For this review, take the finished solid that the model builds, in its own axes (mm). Give positions to 0.01 mm unless a question says otherwise; leave off trailing zeros. Write each loop counter-clockwise with the first axis right and the second up, starting at its lowest first coordinate (ties: lowest second). Pieces come first, ordered by that corner, then holes. Notation, with made-up numbers: M 54.5,60 L 75.5,60 A28 ccw 75.5,87 Z; hole C -6,17.25 d2. An arc over 180 degrees is marked long. Write item = value, one per line.
```python
from build123d import *

# Parameters (mm, degrees)
SKETCH1_R           = 3
SKETCH1_R_2         = 1.5
BOSS_EXTRUDE1_DEPTH = 4


with BuildPart() as part:
    # Sketch1 → Boss-Extrude1 (new body)
    with BuildSketch(Plane.XY):
        with BuildLine():
            Line((2, 13), (2.375498971, 4.399659605))
            ThreePointArc((2.375498971, 4.399659605), (3.535533906, 3.535533906), (4.399659605, 2.375498971))
            Line((4.399659605, 2.375498971), (13, 2))
            ThreePointArc((13, 2), (15, 0), (13, -2))
            Line((13, -2), (4.399659605, -2.375498971))
            ThreePointArc((4.399659605, -2.375498971), (3.535533906, -3.535533906), (2.375498971, -4.399659605))
            Line((2.375498971, -4.399659605), (2, -13))
            ThreePointArc((2, -13), (0, -15), (-2, -13))
            Line((-2, -13), (-2.375498971, -4.399659605))
            ThreePointArc((-2.375498971, -4.399659605), (-3.535533906, -3.535533906), (-4.399659605, -2.375498971))
            Line((-4.399659605, -2.375498971), (-13, -2))
            ThreePointArc((-13, -2), (-15, 0), (-13, 2))
            Line((-13, 2), (-4.399659605, 2.375498971))
            ThreePointArc((-4.399659605, 2.375498971), (-3.535533906, 3.535533906), (-2.375498971, 4.399659605))
            Line((-2.375498971, 4.399659605), (-2, 13))
            ThreePointArc((-2, 13), (0, 15), (2, 13))
        make_face()
        Circle(SKETCH1_R, mode=Mode.SUBTRACT)
        with Locations((0, 13)):
            Circle(SKETCH1_R_2, mode=Mode.SUBTRACT)
        with Locations((13, 0)):
            Circle(SKETCH1_R_2, mode=Mode.SUBTRACT)
        with Locations((0, -13)):
            Circle(SKETCH1_R_2, mode=Mode.SUBTRACT)
        with Locations((-13, 0)):
            Circle(SKETCH1_R_2, mode=Mode.SUBTRACT)
    extrude(amount=BOSS_EXTRUDE1_DEPTH)


solid = part.part
```
1. For line 1 along Y through (x, z) = (0, 3); line 2 along Y through (x, z) = (13, 3.15); line 3 along X through (y, z) = (-0.75, 2.55), list the stretches that pass through material, from the lowest coordinate up. Write a range as from..to.
Responses:
line_1 = -15..-14.5, -11.5..-3, 3..11.5, 14.5..15
line_2 = -2..-1.5, 1.5..2
line_3 = -14.85..-14.3, -11.7..-2.9, 2.9..11.7, 14.3..14.85
2. We need section D-D, the plane y = -7. Write out the cut boundary in (x, z).
Responses:
outline = M -2.26,0 L 2.26,0 L 2.26,4 L -2.26,4 Z
3. Insertion check: P1, Ø1.8, axis at x = 0, y = 13, coming from the +Z side; P2, Ø1.5, axis at x = -9.5, z = 2.5, coming from the +Y side; P3, Ø2, axis at y = -7.5, z = 1, coming from the -X side. Each pin has a flat end and moves straight along its axis. Give the tip position at first contact, or say it passes through.
Responses:
P1 = through
P2 = 2.19
P3 = -2.28
4. We need section B-B, the plane z = 2.4. Write out the cut boundary in (x, y).
Responses:
outline = M -13,-2 L -4.4,-2.38 A5 ccw -2.38,-4.4 L -2,-13 A2 ccw 2,-13 L 2.38,-4.4 A5 ccw 4.4,-2.38 L 13,-2 A2 ccw 13,2 L 4.4,2.38 A5 ccw 2.38,4.4 L 2,13 A2 ccw -2,13 L -2.38,4.4 A5 ccw -4.4,2.38 L -13,2 A2 ccw Z; hole C -13,0 d3; hole C 0,0 d6; hole C 0,-13 d3; hole C 0,13 d3; hole C 13,0 d3
5. We need section A-A, the plane y = 0. Write out the cut boundary in (x, z), then the cut area to 3 significant figures.
Responses:
outline = M -15,0 L -14.5,0 L -14.5,4 L -15,4 Z; M -11.5,0 L -3,0 L -3,4 L -11.5,4 Z; M 3,0 L 11.5,0 L 11.5,4 L 3,4 Z; M 14.5,0 L 15,0 L 15,4 L 14.5,4 Z
area = 72.0 mm2
6. The part is to be moulded in two halves that separate along Y. For faces 1 (the face through (2.3, -2.2, 0)), 2 (the face through (-0.325, 11.536, 1.972)), 3 (the face through (-3.55, 3.52, 1.97)), say which applies: +Y half, -Y half, draft (parallel to the pull), parting line (faces both ways), or undercut.
Responses:
face_1 = draft
face_2 = undercut
face_3 = +Y half
